Build history of the part. All positions in model axes, mm. Give positions to 0.01 mm unless a question says otherwise; leave off trailing zeros. Write each loop counter-clockwise with the first axis right and the second up, starting at its lowest first coordinate (ties: lowest second). Pieces come first, ordered by that corner, then holes. Notation, with made-up numbers: (77.5, -32) - (115.5, -32) arc R25 ccw to (115.5, -7) - close; hole circle Ø8 at (10, 8). An arc over 180 degrees is marked (long way). Use one line per item in the form item = value. Start each with the question number.
from build123d import *

# Parameters (mm, degrees)
F0_R     = 6
F0_R_2   = 1.6
F1_DEPTH = 1.5


with BuildPart() as f1:
    # F0 (on Front) → F1 (new body)
    with BuildSketch(Plane.XZ):
        with BuildLine():
            ThreePointArc((31.112698, 16.970563), (31.112698, 31.112698), (16.970563, 31.112698))
            Line((16.970563, 31.112698), (13.300916, 27.844789))
            ThreePointArc((13.300916, 27.844789), (0, 22.78084), (-13.300916, 27.844789))
            Line((-13.300916, 27.844789), (-16.970563, 31.112698))
            ThreePointArc((-16.970563, 31.112698), (-31.112698, 31.112698), (-31.112698, 16.970563))
            Line((-31.112698, 16.970563), (-30.529389, 16.12375))
            ThreePointArc((-30.529389, 16.12375), (-27.90272, 10.719178), (-27, 4.778312))
            Line((-27, 4.778312), (-27, -4.778312))
            ThreePointArc((-27, -4.778312), (-27.90272, -10.719178), (-30.529389, -16.12375))
            Line((-30.529389, -16.12375), (-31.112698, -16.970563))
            ThreePointArc((-31.112698, -16.970563), (-31.112698, -31.112698), (-16.970563, -31.112698))
            Line((-16.970563, -31.112698), (-13.300916, -27.844789))
            ThreePointArc((-13.300916, -27.844789), (0, -22.78084), (13.300916, -27.844789))
            Line((13.300916, -27.844789), (16.970563, -31.112698))
            ThreePointArc((16.970563, -31.112698), (31.112698, -31.112698), (31.112698, -16.970563))
            Line((31.112698, -16.970563), (30.529389, -16.12375))
            ThreePointArc((30.529389, -16.12375), (27.90272, -10.719178), (27, -4.778312))
            Line((27, -4.778312), (27, 4.778312))
            ThreePointArc((27, 4.778312), (27.90272, 10.719178), (30.529389, 16.12375))
            Line((30.529389, 16.12375), (31.112698, 16.970563))
        make_face()
        Circle(F0_R, mode=Mode.SUBTRACT)
        with Locations((15.25, 15.25)):
            Circle(F0_R_2, mode=Mode.SUBTRACT)
    extrude(amount=F1_DEPTH)


solid = f1.part
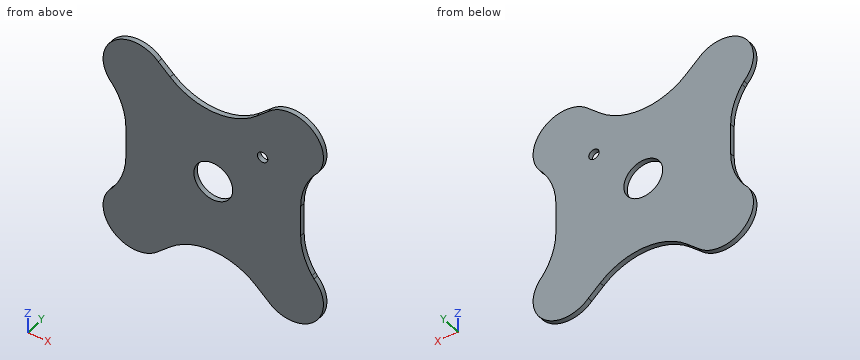
(1) Cut at B-B, the plane x = 0. Give the cut face in (y, z).
(2) Cut at D-D, the plane x = -7. Give the cut face in (y, z), then the cut area to 3 significant figures.
(3) Cut at A-A, the plane z = 0. Give the cut face in (x, y).
(4) Wall check: line 1 (Z direction, x = 0, y = -0.7); line 2 (Z direction, x = 15, y = -0.8); line 3 (X direction, y = -0.45, z = 16). Give the ranges that are in metal, low to high. Write a range as from..to.
Solution:
q1.outline = (-1.5, -22.78) - (0, -22.78) - (0, -6) - (-1.5, -6) - close; (-1.5, 6) - (0, 6) - (0, 22.78) - (-1.5, 22.78) - close
q2.outline = (-1.5, -24.05) - (0, -24.05) - (0, 24.05) - (-1.5, 24.05) - close
q2.area = 72.1 mm2
q3.outline = (-27, -1.5) - (-6, -1.5) - (-6, 0) - (-27, 0) - close; (6, -1.5) - (27, -1.5) - (27, 0) - (6, 0) - close
q4.line_1 = -22.78..-6, 6..22.78
q4.line_2 = -29.36..13.67, 16.83..29.36
q4.line_3 = -30.44..13.84, 16.66..30.44
